```python
from build123d import *

# Parameters (mm, degrees)
SKETCH1_W          = 15.875
SKETCH1_H          = 254
SKETCH2_W          = 19.05
SKETCH2_H          = 19.05
CUT_EXTRUDE1_DEPTH = 255.990257167


with BuildPart() as part:
    # Sketch1 → Revolve1 (revolve)
    with BuildSketch(Plane(origin=(0, 0, 0), x_dir=(1, 0, 0), z_dir=(0, 1, 0))):
        with Locations((-7.9375, -127)):
            Rectangle(SKETCH1_W, SKETCH1_H)
    revolve(axis=Axis((0, 0, 0), (0, 0, 1)))

    # Sketch2 → Cut-Extrude1 (cut, through all)
    with BuildSketch(Plane.XY.offset(254)):
        Rectangle(SKETCH2_W, SKETCH2_H)
    extrude(amount=-CUT_EXTRUDE1_DEPTH, mode=Mode.SUBTRACT)


solid = part.part
```
For this review, take the finished solid that the model builds, in its own axes (mm). A direction names the side the tool comes from. Round coordinates to 2 decimals unless told otherwise and drop trailing zeros. Order: outer loops, then holes, each group sorted by start corner. A loop starts at its lowest first (then second) coordinate and runs counter-clockwise, first axis right, second up.
Q1. Wall thickness on line 1 (X direction, y = 0.5, z = 155) (3 decimals); line 2 (X direction, y = 1, z = 49) (3 decimals): over which ranges is each line inside the solid? List them lowest first.
Findings below:
line 1: x = -15.867 to -9.525, 9.525 to 15.867
line 2: x = -15.843 to -9.525, 9.525 to 15.843
Q2. Mouldability with a two-part tool opening along X and no side actions: class faces 1 (the flat face through (9.525, 0, 129)), 2 (the cylindrical face through (3.441, 15.497, 125.222)), 3 (the flat face through (-10, 0, 0)) as pulls with the +X half, pulls with the -X half, needs draft (parallel to the pull), parting line crosses it, or undercut.
Findings below:
face 1: undercut
face 2: parting line crosses it
face 3: needs draft
Q3. We need section C-C, the plane z = 47. Give the boundary of the cut face in (x, y) (3 decimals), plus the area to 3 significant figures.
Findings below:
outline: circle Ø31.75 at (0, 0); hole (-9.525, -9.525) - (9.525, -9.525) - (9.525, 9.525) - (-9.525, 9.525) - close
area: 429 mm2
Q4. Insertion check: P1, Ø1.5, axis at x = 7, z = 50.5, coming from the +Y side; P2, Ø12, axis at x = 7, z = 124.5, coming from the +Y side; P3, Ø2, axis at x = 7.5, z = 66, coming from the -Y side. Each pin has a flat end and moves straight along its axis. Give the tip position at first contact, or say it passes through.
Findings below:
P1: stops at y = 14.59
P2: stops at y = 15.84
P3: stops at y = -14.48
Q5. Machinability: for faces 4 (the flat face through (-9.525, 0, 129)), 5 (the flat face through (-10, 0, 254)), which of the approach directions +Z, -Z, +X, -X, +Y, -Y give a long, thin tool a straight path to every point of the face, cutting with its end or side? Answer none if there is none.
Findings below:
face 4: +Z, -Z
face 5: +Z, +X, -X, +Y, -Y
Q6. We need section A-A, the plane x = 0. Give the boundary of the cut face in (y, z) (3 decimals), plus the area to 3 significant figures.
Findings below:
outline: (-15.875, 0) - (-9.525, 0) - (-9.525, 254) - (-15.875, 254) - close; (9.525, 0) - (15.875, 0) - (15.875, 254) - (9.525, 254) - close
area: 3,230 mm2
